Verification items for the finished model (mm, model axes). A direction names the side the tool comes from. Give positions to 0.01 mm unless a question says otherwise; leave off trailing zeros. Loops run counter-clockwise (first coordinate to the right, second up) from the corner with the lowest first, then second, coordinate; pieces in that order, holes last. Notation, with made-up numbers: (19, 55.5) - (41, 55.5) arc R15 cw to (41, 74.5) - close; hole circle Ø6 at (47, 49.5). An arc over 180 degrees is marked (long way). Put each result on its own line as item: value. Start each with the question number.
```python
from build123d import *

# Parameters (mm, degrees)
SKETCH1_R                       = 3.175
BOSS_EXTRUDE1_DEPTH             = 127
CUT_EXTRUDE2_DEPTH              = 3.175
F_32_0_116_DIAMETER_HOLE1_D     = 2.9464
F_32_0_116_DIAMETER_HOLE1_DEPTH = 25.4
F_32_0_116_DIAMETER_HOLE1_TIP   = 0.885187864
SKETCH7_R                       = 0.79375
CUT_EXTRUDE3_DEPTH              = 5.08
SKETCH10_W                      = 3.175
SKETCH10_H                      = 1.5875
CUT_EXTRUDE4_DEPTH              = 5.715
LPATTERN1_COUNT                 = 4
LPATTERN1_PITCH                 = 12.7


with BuildPart() as part:
    # Sketch1 → Boss-Extrude1 (new body)
    with BuildSketch(Plane(origin=(0, 0, 0), x_dir=(0, 0, -1), z_dir=(1, 0, 0))):
        Circle(SKETCH1_R)
    extrude(amount=BOSS_EXTRUDE1_DEPTH)

    # Sketch2 → Revolve1 (revolve)
    with BuildSketch(Plane.XY, mode=Mode.PRIVATE) as revolve1_sk:
        with BuildLine():
            Line((142.875, 0), (79.375, 0))
            Line((79.375, 0), (79.375, 5.207))
            Line((79.375, 5.207), (136.628717025, 5.207))
            ThreePointArc((136.628717025, 5.207), (140.694700916, 3.73452755), (142.875, 0))
        make_face()
    revolve(revolve1_sk.sketch.rotate(Axis((127, 0, 0), (-1, 0, 0)), 90), axis=Axis((127, 0, 0), (-1, 0, 0)))

    # Sketch4 → Cut-Extrude2 (cut)
    with BuildSketch(Plane(origin=(0, 0, 0), x_dir=(1, 0, 0), z_dir=(0, 1, 0))):
        with BuildLine():
            Line((76.2, 1.671783879), (66.675, 1.671783879))
            ThreePointArc((66.675, 1.671783879), (65.041030381, 0.03781426), (66.675, -1.596155359))
            Line((66.675, -1.596155359), (76.2, -1.596155359))
            ThreePointArc((76.2, -1.596155359), (77.833969619, 0.03781426), (76.2, 1.671783879))
        make_face()
    extrude(amount=CUT_EXTRUDE2_DEPTH, mode=Mode.SUBTRACT)

    # 32 _0.116_ Diameter Hole1
    with Locations(Plane(origin=(0, 0, 0), x_dir=(-1, 0, 0), z_dir=(0, 1, 0))):
        with Locations((-71.4375, -0.084283879)):
            Hole(F_32_0_116_DIAMETER_HOLE1_D / 2, depth=F_32_0_116_DIAMETER_HOLE1_DEPTH)
            with Locations((0, 0, -(F_32_0_116_DIAMETER_HOLE1_DEPTH + F_32_0_116_DIAMETER_HOLE1_TIP / 2))):  # 118° drill point
                Cone(0, F_32_0_116_DIAMETER_HOLE1_D / 2, F_32_0_116_DIAMETER_HOLE1_TIP, mode=Mode.SUBTRACT)

    # Sketch7 → Cut-Extrude3 (cut, symmetric)
    with BuildSketch(Plane.XY):
        with Locations(Location((12.7, 1.27, 0), (0, 0, 180))):
            Circle(SKETCH7_R)
    cut_extrude3 = extrude(amount=CUT_EXTRUDE3_DEPTH, both=True, mode=Mode.SUBTRACT)

    # Sketch10 → Cut-Extrude4 (cut)
    with BuildSketch(Plane(origin=(0, 0, 0), x_dir=(1, 0, 0), z_dir=(0, 1, 0))):
        with Locations((12.7, 0)):
            Rectangle(SKETCH10_W, SKETCH10_H)
    cut_extrude4 = extrude(amount=CUT_EXTRUDE4_DEPTH, mode=Mode.SUBTRACT)

    # LPattern1: Cut-Extrude3, Cut-Extrude4 ×4
    with Locations(*[(i * LPATTERN1_PITCH, 0, 0) for i in range(1, LPATTERN1_COUNT)]):
        add(cut_extrude3, mode=Mode.SUBTRACT)
        add(cut_extrude4, mode=Mode.SUBTRACT)


solid = part.part
```
1) Depth check by flat-ended pin: P1, Ø6, axis at y = 3, z = -3, coming from the -X side; P2, Ø0.9, axis at x = 51.5, y = 1.5, coming from the -Z side; P3, Ø3.5, axis at x = 25, y = 2, coming from the -Z side; P4, Ø6, axis at y = 1, z = 3.5, coming from the +X side. Enter the tip coordinate at first touch or a pass-through.
2) Draft check along X on faces 1 (the face through (108.403, -1.564, -4.967)), 2 (the face through (0, 0, 0)), 3 (the face through (51.1, 2.2, -0.794)). Enter one of: pulls with the +X half, pulls with the -X half, needs draft (parallel to the pull), parting line crosses it, or undercut.
3) Section check A-A, the plane x = 115. Enter the section's corners in (y, z).
4) Section check B-B, the plane x = 55. Enter the section's corners in (y, z) (3 decimals), plus the area to 3 significant figures.
5) Scan lines: line 1 along X through (y, z) = (1.27, 2.1); line 2 along X through (y, z) = (1.27, 1.7); line 3 along Y through (x, z) = (25.4, -2.2). Record each from-to range of solid material in increasing order. Write a range as from..to.
6) Set-up check for faces 4 (the face through (72.229, -1.612, 1.158)), 5 (the face through (26, 2, -0.794)), 6 (the face through (39.13, -3.1, 0.69)): record each of +Z, -Z, +X, -X, +Y, -Y from which the full face is reachable in a straight line by a thin tool's end or side.
Results are:
1. P1: stops at x = 0
1. P2: stops at z = -2.99
1. P3: stops at z = -3.17
1. P4: stops at x = 142.72
2. face 1: needs draft
2. face 2: pulls with the -X half
2. face 3: undercut
3. outline: circle Ø10.41 at (0, 0)
4. outline: circle Ø6.35 at (0, 0)
4. area: 31.7 mm2
5. line 1: x = 0..11.91, 13.49..24.61, 26.19..37.31, 38.89..50.01, 51.59..141.86
5. line 2: x = 0..11.91, 13.49..24.61, 26.19..37.31, 38.89..50.01, 51.59..142.08
5. line 3: y = -2.29..0.48, 2.06..2.29
6. face 4: +Y, -Y
6. face 5: +Y
6. face 6: -X
